```python
from build123d import *

# Parameters (mm, degrees)
SCHIZZO1_W                   = 130
SCHIZZO1_H                   = 130
ESTRUSIONE_ESTRUSIONE1_DEPTH = 6
SCHIZZO2_W                   = 70
SCHIZZO2_H                   = 60
TAGLIO_ESTRUSIONE1_DEPTH     = 15
SCHIZZO3_R                   = 8
TAGLIO_ESTRUSIONE2_DEPTH     = 15
SCHIZZO4_W                   = 30
SCHIZZO4_H                   = 15
TAGLIO_ESTRUSIONE3_DEPTH     = 15


with BuildPart() as part:
    # Schizzo1 → Estrusione-Estrusione1 (new body)
    with BuildSketch(Plane.XY):
        Rectangle(SCHIZZO1_W, SCHIZZO1_H)
    extrude(amount=ESTRUSIONE_ESTRUSIONE1_DEPTH)

    # Schizzo2 → Taglio-Estrusione1 (cut)
    with BuildSketch(Plane.XY.offset(6)):
        with Locations((0, 12)):
            Rectangle(SCHIZZO2_W, SCHIZZO2_H)
    extrude(amount=-TAGLIO_ESTRUSIONE1_DEPTH, mode=Mode.SUBTRACT)

    # Schizzo3 → Taglio-Estrusione2 (cut)
    with BuildSketch(Plane.XY.offset(6)):
        with Locations((0, -34)):
            Circle(SCHIZZO3_R)
    extrude(amount=-TAGLIO_ESTRUSIONE2_DEPTH, mode=Mode.SUBTRACT)

    # Schizzo4 → Taglio-Estrusione3 (cut)
    with BuildSketch(Plane.XY.offset(6)):
        with Locations((-50, 24.5)):
            Rectangle(SCHIZZO4_W, SCHIZZO4_H)
    extrude(amount=-TAGLIO_ESTRUSIONE3_DEPTH, mode=Mode.SUBTRACT)


solid = part.part
```
Verification items for the finished model (mm, model axes). A direction names the side the tool comes from. Round coordinates to 2 decimals unless told otherwise and drop trailing zeros. Order: outer loops, then holes, each group sorted by start corner. A loop starts at its lowest first (then second) coordinate and runs counter-clockwise, first axis right, second up.
1) Cross-section at B-B, the plane y = -34. Record the cut outline in (x, z), plus the area to 3 significant figures.
Geometry says:
outline: (-65, 0) - (-8, 0) - (-8, 6) - (-65, 6) - close; (8, 0) - (65, 0) - (65, 6) - (8, 6) - close
area: 684 mm2
2) Cross-section at C-C, the plane x = 0. Record the cut outline in (y, z), plus the area to 3 significant figures.
Geometry says:
outline: (-65, 0) - (-42, 0) - (-42, 6) - (-65, 6) - close; (-26, 0) - (-18, 0) - (-18, 6) - (-26, 6) - close; (42, 0) - (65, 0) - (65, 6) - (42, 6) - close
area: 324 mm2
3) Draft check along Y on faces 4 (the flat face through (-1, 65, 3)), 5 (the flat face through (0, 42, 3)), 6 (the flat face through (14, -28, 0)). Enter one of: +Y half, -Y half, draft (parallel to the pull), parting line (faces both ways), or undercut.
Geometry says:
face 4: +Y half
face 5: undercut
face 6: draft
4) Tool access check on faces 1 (the flat face through (-65, 48, 3)), 2 (the flat face through (-50, 17, 3)), 3 (the flat face through (35, 12, 3)). Record the directions out of +Z, -Z, +X, -X, +Y, -Y that give a thin tool (end or side, any length) a straight path to the whole face; none if there is none.
Geometry says:
face 1: +Z, -Z, -X, +Y, -Y
face 2: +Z, -Z, -X
face 3: +Z, -Z
5) Depth check by flat-ended pin: pin 1 (18.5 mm diameter, centred on x = 0, y = -34, fed in from +Z). Enter the tip coordinate at first touch or a pass-through.
Geometry says:
pin 1: stops at z = 6
6) Material ranges on line 1 (Y direction, x = 0, z = 2.1); line 2 (Y direction, x = -53.5, z = 5.2); line 3 (Y direction, x = -25, z = 5.05), recorded low to high.
Geometry says:
line 1: y = -65 to -42, -26 to -18, 42 to 65
line 2: y = -65 to 17, 32 to 65
line 3: y = -65 to -18, 42 to 65
7) Cross-section at A-A, the plane x = -43. Record the cut outline in (y, z).
Geometry says:
outline: (-65, 0) - (17, 0) - (17, 6) - (-65, 6) - close; (32, 0) - (65, 0) - (65, 6) - (32, 6) - close
